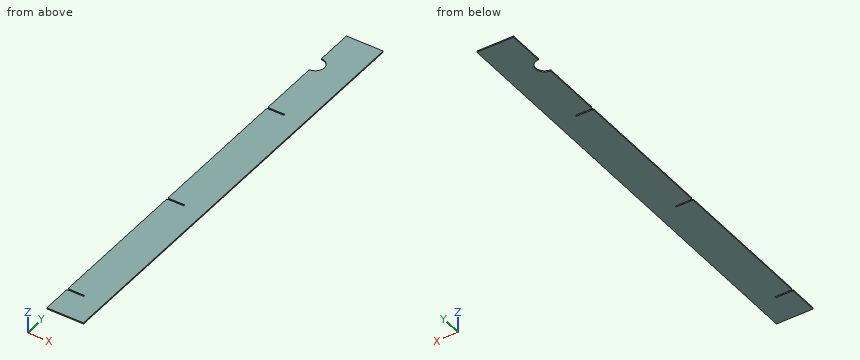
Autodesk Inventor part; units mm, degrees
ref_plane "YZ Plane" through (0, 0, 0) normal (1, 0, 0) x (0, 1, 0)
ref_plane "XZ Plane" through (0, 0, 0) normal (0, 1, 0) x (-1, 0, 0)
ref_plane "XY Plane" through (0, 0, 0) normal (0, 0, 1) x (1, 0, 0)
sketch "Sketch1" plane through (0, 0, 0) normal (0, 0, 1) x (1, 0, 0)
  line L0 (0, 1489.5) -> (-122.6558, 1489.5)
  line L1 (-122.6558, 1489.5) -> (-122.6558, 0)
  line L2 (-122.6558, 0) -> (0, 0)
  line L3 (0, 0) -> (0, 1489.5)
  line L4 (-122.6558, 100) -> (-66, 100)
  line L5 (-66, 100) -> (-66, 105)
  line L6 (-66, 105) -> (-122.6558, 105)
  line L7 (-122.6558, 105) -> (-122.6558, 100)
  line L8 (-122.6558, 596.6667) -> (-66, 596.6667)
  line L9 (-66, 596.6667) -> (-66, 601.6667)
  line L10 (-66, 601.6667) -> (-122.6558, 601.6667)
  line L11 (-122.6558, 601.6667) -> (-122.6558, 596.6667)
  line L12 (-122.6558, 1093.3333) -> (-66, 1093.3333)
  line L13 (-66, 1093.3333) -> (-66, 1098.3333)
  line L14 (-66, 1098.3333) -> (-122.6558, 1098.3333)
  line L15 (-122.6558, 1098.3333) -> (-122.6558, 1093.3333)
  circle A0 centre (-122.6558, 1335) radius 30
  point P0 (-122.6558, 601.6667)
  point P1 (-122.6558, 1365)
  point P2 (-122.6558, 1305)
  dimension "d0" = 1489.5
  dimension "d1" = 122.6559
  dimension "d2" = 5
  dimension "d4" = 100
  dimension "d7" = 496.6667
  dimension "d23" = 66
  dimension "d29" = 60
  dimension "d30" = 1335
extrude "Plate1" add sketch "Sketch1" along normal blind 4 contours L3 L2 L1 L4 L5 L6 L8 L9 L10 L12 L13 L14 A0 L0
chamfer "Corner Chamfer1" distance 3 angle 45 6 edges at (-122.6558, 100, 2) (-122.6558, 105, 2) (-122.6558, 596.6667, 2) (-122.6558, 601.6667, 2) (-122.6558, 1098.3333, 2) (-122.6558, 1093.3333, 2)
equation "\"d0\" = Стрингер_длина"
equation "\"d1\" = стрингер_глубина_7"
equation "\"d2\" = паз_под_стрингер_толщина"
equation "\"d7\" = Шаг_шпангоутов"
equation "\"d23\" = паз_под_стрингер_глубина - Thickness"
equation "\"d29\" = 2 * радиус_выреза_под_сварку"
equation "\"d12\" = Thickness"
equation "\"BendRadius\" = Thickness"
equation "\"BendReliefWidth\" = Thickness"
equation "\"BendReliefDepth\" = 0.5 * Thickness"
equation "\"CornerReliefSize\" = 4 * Thickness"
equation "\"MinimumRemnant\" = 2 * Thickness"
equation "\"TransitionRadius\" = BendRadius"
equation "\"JacobiRadiusSize\" = BendRadius"
equation "\"GapSize\" = Thickness"
properties part number "GBK 3312 stringer 7" material "Steel"
Input: part model. Units: mm. Frame: model coordinates. Coordinates: 2 decimals unless noted, no trailing zeros. Order: outer loops, then holes, each group sorted by start corner. A loop starts at its lowest first (then second) coordinate and runs counter-clockwise, first axis right, second up.
1. Ray query, line 1 along Y through (x, z) = (-89.5, 3.35); line 2 along Y through (x, z) = (-111, 2.25); line 3 along Y through (x, z) = (-95, 2.95). Return the intervals inside material, ascending.
Checked values:
line 1: y = 0 to 100, 105 to 596.67, 601.67 to 1093.33, 1098.33 to 1489.5
line 2: y = 0 to 100, 105 to 596.67, 601.67 to 1093.33, 1098.33 to 1307.36, 1362.64 to 1489.5
line 3: y = 0 to 100, 105 to 596.67, 601.67 to 1093.33, 1098.33 to 1323.37, 1346.63 to 1489.5
2. Cut plane A-A, the plane y = 1335. Return loops of the section in (x, z).
Checked values:
outline: (-92.66, 0) - (0, 0) - (0, 4) - (-92.66, 4) - close
3. Contact query for a flat-ended pin moving along its axis: P1, Ø1.2, axis at y = 101.5, z = 3, coming from the -X side. Output: stop coordinate, or through.
Checked values:
P1: stops at x = -66
